Verification items for the finished model (mm, model axes). Coordinates: 2 decimals unless noted, no trailing zeros. Order: outer loops, then holes, each group sorted by start corner. A loop starts at its lowest first (then second) coordinate and runs counter-clockwise, first axis right, second up. Notation, with made-up numbers: M -24,8.5 L -6,8.5 A37 ccw -6,47.5 Z; hole C -34.75,48 d9. An arc over 180 degrees is marked long. Return JSON: item names as keys, results as strings. Group by question number.
1. Material ranges on line 1 along Y through (x, z) = (7.75, 1.7); line 2 along X through (y, z) = (25, 2.1); line 3 along Y through (x, z) = (-15.5, 0.65), recorded low to high.
2. Section check B-B, the plane x = 15.5. Record the cut outline in (y, z).
3. Section check A-A, the plane y = -29.5. Record the cut outline in (x, z).
4. Gauge pin test, flat ends, axial feed: pin 1 (2.5 mm diameter, centred on x = -7.75, y = -6.58, fed in from -Z); pin 2 (1.5 mm diameter, centred on x = -6, z = 1.5, fed in from -Y); pin 3 (1.5 mm diameter, centred on x = -14.5, z = 1, fed in from +Y); pin 4 (1.5 mm diameter, centred on y = 25.5, z = 1, fed in from -X). Record the tip position at first contact, or that the pin passes through.
5. Section check C-C, the plane z = 0.8. Give the number of separate pieces and of enclosed holes in the cut face, plus the area to 3 significant figures.
```python
from build123d import *

# Parameters (mm, degrees)
ESQUISSE3_W                = 50
ESQUISSE3_H                = 60
BOSS_EXTRU_12_DEPTH        = 3
ESQUISSE4_R                = 1.5
ENL_V_MAT_EXTRU_1_DEPTH    = 5
ESQUISSE6_R                = 6.5
ENL_V_MAT_EXTRU_3_DEPTH    = 10
ESQUISSE7_W                = 5
ESQUISSE7_H                = 10
ESQUISSE7_H_2              = 5
BOSS_EXTRU_13_DEPTH        = 3
R_P_TITION_LIN_AIRE1_COUNT = 5
R_P_TITION_LIN_AIRE1_PITCH = 10


with BuildPart() as part:
    # Esquisse3 → Boss.-Extru.12 (new body)
    with BuildSketch(Plane.XY):
        with Locations((0, -8)):
            Rectangle(ESQUISSE3_W, ESQUISSE3_H)
    extrude(amount=BOSS_EXTRU_12_DEPTH)

    # Esquisse4 → Enlèv. mat.-Extru.1 (cut)
    with BuildSketch(Plane.XY.offset(3)):
        with Locations((-7.75, -6.576606241)):
            Circle(ESQUISSE4_R)
        with Locations((-15.5, -20)):
            Circle(ESQUISSE4_R)
        with Locations((-7.75, -33.423393759)):
            Circle(ESQUISSE4_R)
    enl_v_mat_extru_1 = extrude(amount=-ENL_V_MAT_EXTRU_1_DEPTH, mode=Mode.SUBTRACT)

    # Esquisse6 → Enlèv. mat.-Extru.3 (cut)
    with BuildSketch(Plane.XY.offset(3)):
        with Locations((0, -27)):
            Circle(ESQUISSE6_R)
    extrude(amount=-ENL_V_MAT_EXTRU_3_DEPTH, mode=Mode.SUBTRACT)

    # Symétrie3: Enlèv. mat.-Extru.1 across plane
    add(enl_v_mat_extru_1.mirror(Plane(origin=(0, 0, 0), x_dir=(0, 0, 1), z_dir=(1, 0, 0))), mode=Mode.SUBTRACT)

    # Esquisse7 → Boss.-Extru.13 (add)
    with BuildSketch(Plane.XY.offset(3)):
        with Locations((-20, 27)):
            Rectangle(ESQUISSE7_W, ESQUISSE7_H)
        with Locations((-20, -40.5)):
            Rectangle(ESQUISSE7_W, ESQUISSE7_H_2)
    boss_extru_13 = extrude(amount=-BOSS_EXTRU_13_DEPTH)

    # Répétition linéaire1: Boss.-Extru.13 ×5
    with Locations(*[(i * R_P_TITION_LIN_AIRE1_PITCH, 0, 0) for i in range(1, R_P_TITION_LIN_AIRE1_COUNT)]):
        add(boss_extru_13)


solid = part.part
```
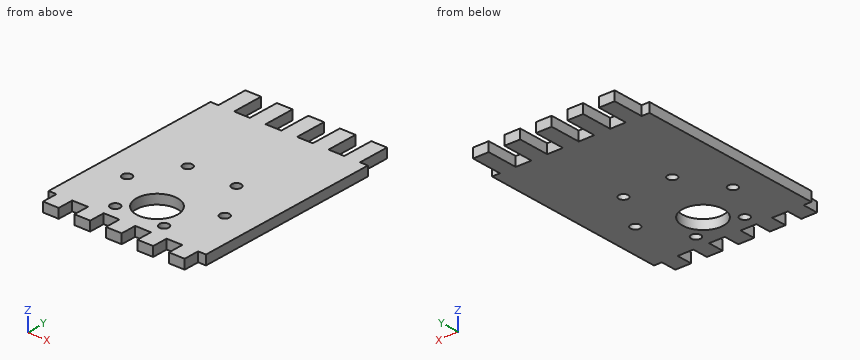
Answers follow:
{
 "1": {"line 1": "-43 to -34.92, -31.92 to -8.08, -5.08 to 32", "line 2": "-22.5 to -17.5, -12.5 to -7.5, -2.5 to 2.5, 7.5 to 12.5, 17.5 to 22.5", "line 3": "-38 to -21.5, -18.5 to 22"},
 "2": {"outline": "M -38,0 L -21.5,0 L -21.5,3 L -38,3 Z; M -18.5,0 L 22,0 L 22,3 L -18.5,3 Z"},
 "3": {"outline": "M -25,0 L -6,0 L -6,3 L -25,3 Z; M 6,0 L 25,0 L 25,3 L 6,3 Z"},
 "4": {"pin 1": "through", "pin 2": "y = -38", "pin 3": "y = 22", "pin 4": "x = -22.5"},
 "5": {"separate pieces": "1", "enclosed holes": "7", "area": "3,200 mm^2"}
}
